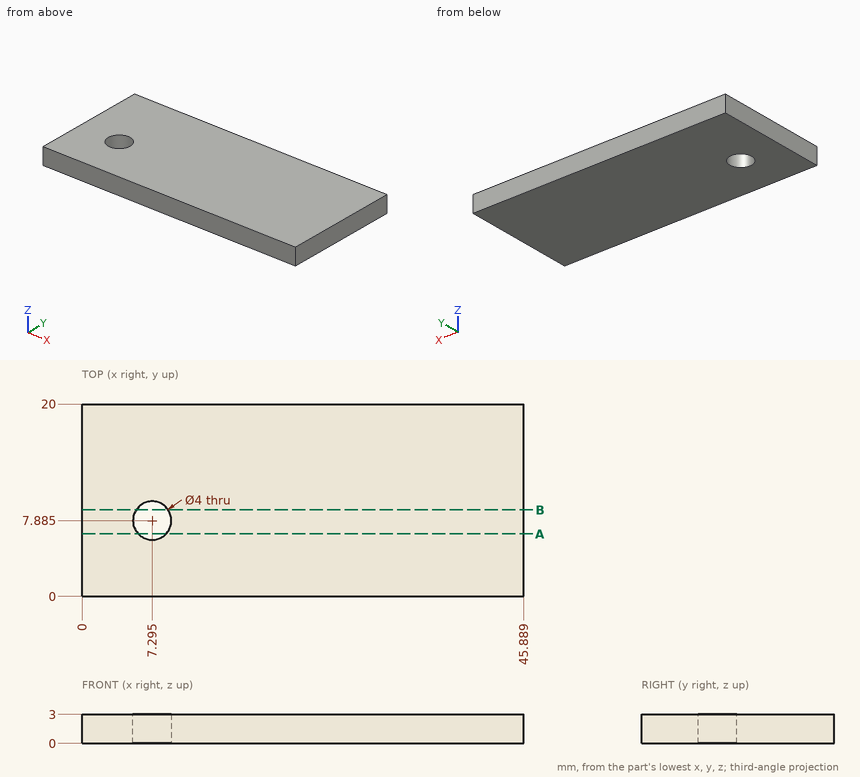
Job drawing, mm, ordinate dimensions from the low corner. One solid piece. Coordinates: 2 decimals unless noted, no trailing zeros. Order: outer loops, then holes, each group sorted by start corner. A loop starts at its lowest first (then second) coordinate and runs counter-clockwise, first axis right, second up. Notation, with made-up numbers: (45, 52) -> (61, 52) arc R36 cw to (61, 86) -> close; hole circle Ø10 at (51.5, -5.5). An arc over 180 degrees is marked (long way). Answer in a Markdown table with one row per item. Add a question column.
Q1. Band-saw the part on B-B, the plane y = 9. List the corners of the cut face in (x, z) (1 decimal), then the cut area to 3 significant figures.
Q2. Wall check: line 1 along X through (y, z) = (8, 2.45); line 2 along X through (y, z) = (9, 1.5) (1 decimal); line 3 along Y through (x, z) = (9, 0.2). Give the ranges that are in metal, low to high. Write a range as [from, to].
Q3. Band-saw the part on A-A, the plane y = 6.5. List the corners of the cut face in (x, z), then the cut area to 3 significant figures.
Answers follow:
| question | item | result |
|---|---|---|
| 1 | outline | (0, 0) -> (5.6, 0) -> (5.6, 3) -> (0, 3) -> close; (9, 0) -> (45.9, 0) -> (45.9, 3) -> (9, 3) -> close |
| 1 | area | 128 mm^2 |
| 2 | line 1 | [0, 5.3], [9.29, 45.89] |
| 2 | line 2 | [0, 5.6], [9, 45.9] |
| 2 | line 3 | [0, 6.84], [8.93, 20] |
| 3 | outline | (0, 0) -> (5.85, 0) -> (5.85, 3) -> (0, 3) -> close; (8.74, 0) -> (45.89, 0) -> (45.89, 3) -> (8.74, 3) -> close |
| 3 | area | 129 mm^2 |
